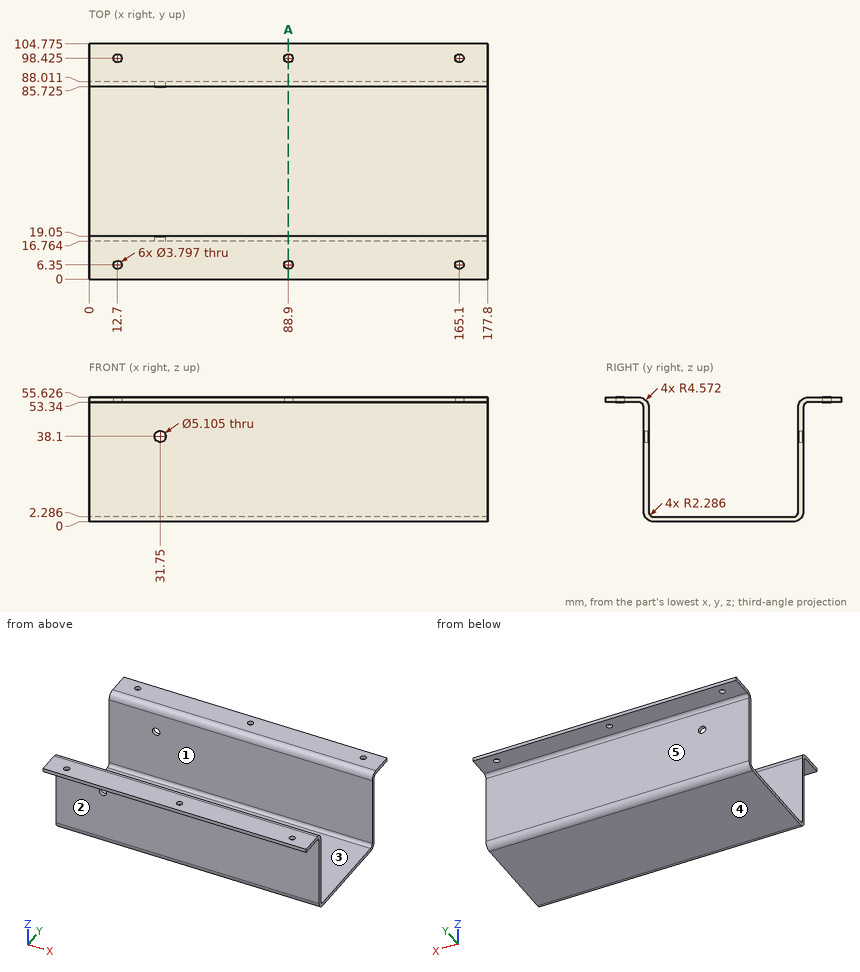
Job drawing, mm, ordinate dimensions from the low corner. One solid piece. A direction names the side the tool comes from. Round coordinates to 2 decimals unless told otherwise and drop trailing zeros. Answer as a JSON object with one key per item and string values.
(1) Band-saw the part on A-A, the plane x = 88.9. Count the separate pieces of the cut face and the enclosed holes in it.
Reported:
{"separate pieces": "3", "enclosed holes": "0"}
(2) Two-plate mould, pull along Y, no slides. Class the marked faces 3, 4 and 5: +Y half, -Y half, draft (parallel to the pull), parting line (faces both ways), or undercut.
Reported:
{"face 3": "undercut", "face 4": "draft", "face 5": "+Y half"}
(3) Pin check, flat tips, straight feed: P1, Ø7, axis at x = 90, y = 8.5, coming from the -Z side; P2, Ø2, axis at x = 151, z = 21.5, coming from the -Y side; P3, Ø6, axis at x = 156, z = 16, coming from the +Y side. Stop position of each tip, or through.
Reported:
{"P1": "stops at z = 53.34", "P2": "stops at y = 16.76", "P3": "stops at y = 88.01"}
(4) Probe probe 1 along Z at (x, y) = (8, 34.5); probe 2 along Y at (x, z) = (12, 54) (1 decimal); probe 3 along Z at (x, y) = (159.5, 96.5). List the from-to ranges inside material, lowest first. Write a range as [from, to].
Reported:
{"probe 1": "z = [0, 2.29]", "probe 2": "y = [0, 4.6], [8.1, 18], [86.8, 96.7], [100.2, 104.8]", "probe 3": "z = [53.34, 55.63]"}
(5) Which spindle directions (+Z, -Z, +X, -X, +Y, -Y) get a long thin tool onto all of the face, cutting with end or side? Do the marked faces 1 and 2. Say none if no direction does.
Reported:
{"face 1": "+Z, +X, -X", "face 2": "-Z, +X, -X, -Y"}
